from build123d import *

# Parameters (mm, degrees)
SKETCH1_W           = 110
SKETCH1_H           = 110
SKETCH1_R           = 2
BOSS_EXTRUDE1_DEPTH = 2
SKETCH3_W           = 10
SKETCH3_H           = 30
BOSS_EXTRUDE2_DEPTH = 45
FILLET1_R           = 15


with BuildPart() as part:
    # Sketch1 → Boss-Extrude1 (new body)
    with BuildSketch(Plane.XY):
        Rectangle(SKETCH1_W, SKETCH1_H)
        with Locations((-50, 50)):
            Circle(SKETCH1_R, mode=Mode.SUBTRACT)
        with Locations((-50, -50)):
            Circle(SKETCH1_R, mode=Mode.SUBTRACT)
        with Locations((50, -50)):
            Circle(SKETCH1_R, mode=Mode.SUBTRACT)
        with Locations((50, 50)):
            Circle(SKETCH1_R, mode=Mode.SUBTRACT)
    extrude(amount=BOSS_EXTRUDE1_DEPTH)

    # Sketch3 → Boss-Extrude2 (add)
    with BuildSketch(Plane(origin=(0, 0, 0), x_dir=(-1, 0, 0), z_dir=(0, 0, -1))):
        Rectangle(SKETCH3_W, SKETCH3_H)
    extrude(amount=BOSS_EXTRUDE2_DEPTH)

    # Fillet1
    fillet1_edges = [part.edges().sort_by_distance(p)[0] for p in [
        (0, -15, -45),
        (0, 15, -45),
    ]]
    fillet(fillet1_edges, radius=FILLET1_R - 0.0001)  # a hair under: the kernel refuses the full size


solid = part.part
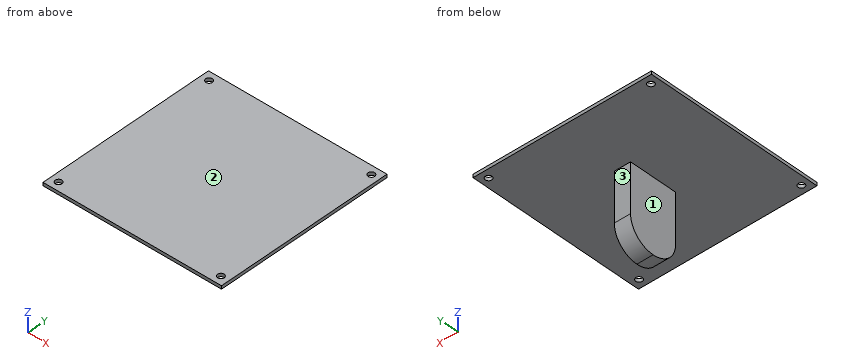
The model under review builds one solid part; all positions refer to its coordinate system, in mm. Face numbers are marked on the shaded views. A direction names the side the tool comes from. Coordinates: 2 decimals unless noted, no trailing zeros. Loops run counter-clockwise (first coordinate to the right, second up) from the corner with the lowest first, then second, coordinate; pieces in that order, holes last. Notation, with made-up numbers: (-24.75, -18.75) -> (22.25, -18.75) arc R30 ccw to (22.25, 9.25) -> close; hole circle Ø10 at (89, 63.25). An arc over 180 degrees is marked (long way). Use a Markdown table: item, result. Add a question column.
1. Add section C-C on z = -13. Write out the cut boundary in (x, y).
2. To check wall thickness, follow line 1 (Y direction, x = 50, z = 0.7); line 2 (Z direction, x = 31.5, y = -6); line 3 (X direction, y = -14.5, z = -1). State the ranges of each line that lie inside material, in increasing order.
3. Add section D-D on y = 17. Write out the cut boundary in (x, z), plus the area to 3 significant figures.
4. Add section A-A on y = -50. Write out the cut boundary in (x, z), plus the area to 3 significant figures.
5. Clearance check with flat-ended pins moving along their axes: pin 1 Ø10 at (x, y) = (0, 13.5) entering from -Z; pin 2 Ø3 at (x, z) = (2, -19.5) entering from +Y; pin 3 Ø24 at (y, z) = (-1, -17) entering from +X. State where each tip first meets the part, or that it passes through.
6. Machinability: for the marked faces 1, 2 and 3, which of the approach directions +Z, -Z, +X, -X, +Y, -Y give a long, thin tool a straight path to every point of the face, cutting with its end or side? Answer none if there is none.
Returned:
| question | item | result |
|---|---|---|
| 1 | outline | (-5, -15) -> (5, -15) -> (5, 15) -> (-5, 15) -> close |
| 2 | line 1 | y = -55 to -52, -48 to 48, 52 to 55 |
| 2 | line 2 | z = 0 to 2 |
| 2 | line 3 | x = -5 to 5 |
| 3 | outline | (-55, 0) -> (55, 0) -> (55, 2) -> (-55, 2) -> close |
| 3 | area | 220 mm² |
| 4 | outline | (-55, 0) -> (-52, 0) -> (-52, 2) -> (-55, 2) -> close; (-48, 0) -> (48, 0) -> (48, 2) -> (-48, 2) -> close; (52, 0) -> (55, 0) -> (55, 2) -> (52, 2) -> close |
| 4 | area | 204 mm² |
| 5 | pin 1 | stops at z = -42.36 |
| 5 | pin 2 | stops at y = 15 |
| 5 | pin 3 | stops at x = 5 |
| 6 | face 1 | -Z, -X, +Y, -Y |
| 6 | face 2 | +Z, +X, -X, +Y, -Y |
| 6 | face 3 | -Z, +X, -X, +Y |
